Work out the finished part from the listing and answer in its coordinate system (mm). A direction names the side the tool comes from. Round coordinates to 2 decimals unless told otherwise and drop trailing zeros. Order: outer loops, then holes, each group sorted by start corner. A loop starts at its lowest first (then second) coordinate and runs counter-clockwise, first axis right, second up. Notation, with made-up numbers: M 63.5,-28.5 L 78.5,-28.5 A24 ccw 78.5,-15.5 Z; hole C 59.25,-17.75 d3. An arc over 180 degrees is marked long. Return JSON: item names as keys, results as strings.
from build123d import *

# Parameters (mm, degrees)
F0_W     = 10
F0_H     = 5
F1_DEPTH = 1
F3_DEPTH = 7
F5_D     = 1
F5_DEPTH = 1


with BuildPart() as f1:
    # F0 (on Front) → F1 (new body)
    with BuildSketch(Plane.XZ):
        with Locations((49.226046, 17.170396)):
            Rectangle(F0_W, F0_H)
        Polygon((39.226046, 4.670396), (59.226046, 4.670396), (59.226046, 14.670396), (54.226046, 14.670396), (44.226046, 14.670396), (39.226046, 14.670396), align=None)
    extrude(amount=-F1_DEPTH)

    # F2 (on face) → F3 (join)
    with BuildSketch(Plane(origin=(0, 1, 0), x_dir=(-1, 0, 0), z_dir=(0, 1, 0))):
        Polygon((-59.226046, 14.670396), (-59.226046, 4.670396), (-39.226046, 4.670396), (-39.226046, 14.670396), (-44.226046, 14.670396), (-44.226046, 19.670396), (-54.226046, 19.670396), (-54.226046, 14.670396), align=None)
        Polygon((-58.226046, 5.670396), (-58.226046, 13.670396), (-53.226046, 13.670396), (-53.226046, 18.670396), (-45.226046, 18.670396), (-45.226046, 13.670396), (-40.226046, 13.670396), (-40.226046, 5.670396), align=None, mode=Mode.SUBTRACT)
    extrude(amount=F3_DEPTH)

    # F5
    with Locations(Plane.XY.offset(19.670396)):
        with Locations((46.226046, 2.054661), (52.226046, 2.061454)):
            Hole(F5_D / 2, depth=F5_DEPTH)


solid = f1.part
Item 1: Each of these flat-tipped pins is pushed along its axis until it touches: pin 1 (6 mm diameter, centred on x = 47.5, z = 6.5, fed in from -Y); pin 2 (2.5 mm diameter, centred on y = 4, z = 16, fed in from -X); pin 3 (1.5 mm diameter, centred on x = 41, y = 2.5, fed in from +Z); pin 4 (1.5 mm diameter, centred on y = 5, z = 16, fed in from +X). Where does it stop, or does it pass through?
Output:
{"pin 1": "stops at y = 0", "pin 2": "stops at x = 44.23", "pin 3": "stops at z = 14.67", "pin 4": "stops at x = 54.23"}
Item 2: Find section B-B (x = 48.5). Determine the outline of the cut face in (y, z).
Output:
{"outline": "M 0,4.67 L 8,4.67 L 8,5.67 L 1,5.67 L 1,18.67 L 8,18.67 L 8,19.67 L 0,19.67 Z"}
Item 3: Consider line 1 along Z through (x, y) = (50.75, 5.75); line 2 along Z through (x, y) = (57.25, 4.5); line 3 along X through (y, z) = (7, 6.75). Determine where each line is inside the solid, lowest interval first. Write a range as [from, to].
Output:
{"line 1": "z = [4.67, 5.67], [18.67, 19.67]", "line 2": "z = [4.67, 5.67], [13.67, 14.67]", "line 3": "x = [39.23, 40.23], [58.23, 59.23]"}
Item 4: The mould has two halves that part along Y. Classify faces 4 (the flat face through (49, 0, 11)), 5 (the cylindrical face through (51.764, 1.87, 19.163)), 6 (the flat face through (59.226, 4, 10)): pulls with the +Y half, pulls with the -Y half, needs draft (parallel to the pull), parting line crosses it, or undercut.
Output:
{"face 4": "pulls with the -Y half", "face 5": "undercut", "face 6": "needs draft"}
Item 5: Find section A-A (z = 12). Determine the outline of the cut face in (x, y).
Output:
{"outline": "M 39.23,0 L 59.23,0 L 59.23,8 L 58.23,8 L 58.23,1 L 40.23,1 L 40.23,8 L 39.23,8 Z"}
Item 6: Which of the six approach directions +Z, -Z, +X, -X, +Y, -Y give full straight-line access (tool end or side, diameter ignored) to faces 1 (the flat face through (58.226, 4, 10)), 2 (the flat face through (57, 4, 14.67)), 3 (the flat face through (42, 4, 14.67))?
Output:
{"face 1": "+Y", "face 2": "+Z, +X, +Y, -Y", "face 3": "+Z, -X, +Y, -Y"}
Item 7: Find section C-C (y = 3.25). Determine the outline of the cut face in (x, z).
Output:
{"outline": "M 39.23,4.67 L 59.23,4.67 L 59.23,14.67 L 54.23,14.67 L 54.23,19.67 L 44.23,19.67 L 44.23,14.67 L 39.23,14.67 Z; hole M 40.23,5.67 L 58.23,5.67 L 58.23,13.67 L 53.23,13.67 L 53.23,18.67 L 45.23,18.67 L 45.23,13.67 L 40.23,13.67 Z"}
